Autodesk Inventor part; units mm, degrees
ref_plane "YZ Plane" through (0, 0, 0) normal (1, 0, 0) x (0, 1, 0)
ref_plane "XZ Plane" through (0, 0, 0) normal (0, 1, 0) x (-1, 0, 0)
ref_plane "XY Plane" through (0, 0, 0) normal (0, 0, 1) x (1, 0, 0)
sketch "Sketch1" plane through (0, 0, 0) normal (0, 0, 1) x (1, 0, 0)
  circle A0 centre (0, 0) radius 51
  dimension "d0" = 102
extrude "Extrusion1" add sketch "Sketch1" along normal blind 5
sketch "Sketch2" plane through (0, 0, 5) normal (0, 0, 1) x (1, 0, 0)
  point P0 (0, 0)
  point P1 (0, 0)
hole "Hole1" at (0, 0, 5) direction (0, 0, -1) diameter 6.6 depth 8 tip angle 118
sketch "Sketch3" plane through (0, 0, 5) normal (0, 0, 1) x (1, 0, 0)
  circle A0 centre (0, 0) radius 15 construction
  point P0 (-15, 0)
  point P1 (0, 15)
  point P2 (15, 0)
  point P3 (0, -15)
  dimension "d10" = 30
hole "Hole2" at (-15, 0, 5) at (0, 15, 5) at (15, 0, 5) at (0, -15, 5) direction (0, 0, -1) diameter 3.4 depth 8 tip angle 118
sketch "Sketch4" plane through (0, 0, 5) normal (0, 0, 1) x (1, 0, 0)
  line L0 (-51, 1.6) -> (-51, -1.6)
  line L1 (-51, -1.6) -> (-46, -1.6)
  line L2 (-46, -1.6) -> (-46, -2.75)
  line L3 (-46, -2.75) -> (-43.6, -2.75)
  line L4 (-43.6, -2.75) -> (-43.6, 2.75)
  line L5 (-43.6, 2.75) -> (-46, 2.75)
  line L6 (-46, 2.75) -> (-46, 1.6)
  line L7 (-46, 1.6) -> (-51, 1.6)
  line L8 (-1.6, -51) -> (1.6, -51)
  line L9 (1.6, -51) -> (1.6, -46)
  line L10 (1.6, -46) -> (2.75, -46)
  line L11 (2.75, -46) -> (2.75, -43.6)
  line L12 (2.75, -43.6) -> (-2.75, -43.6)
  line L13 (-2.75, -43.6) -> (-2.75, -46)
  line L14 (-2.75, -46) -> (-1.6, -46)
  line L15 (-1.6, -46) -> (-1.6, -51)
  line L16 (51, -1.6) -> (51, 1.6)
  line L17 (51, 1.6) -> (46, 1.6)
  line L18 (46, 1.6) -> (46, 2.75)
  line L19 (46, 2.75) -> (43.6, 2.75)
  line L20 (43.6, 2.75) -> (43.6, -2.75)
  line L21 (43.6, -2.75) -> (46, -2.75)
  line L22 (46, -2.75) -> (46, -1.6)
  line L23 (46, -1.6) -> (51, -1.6)
  line L24 (1.6, 51) -> (-1.6, 51)
  line L25 (-1.6, 51) -> (-1.6, 46)
  line L26 (-1.6, 46) -> (-2.75, 46)
  line L27 (-2.75, 46) -> (-2.75, 43.6)
  line L28 (-2.75, 43.6) -> (2.75, 43.6)
  line L29 (2.75, 43.6) -> (2.75, 46)
  line L30 (2.75, 46) -> (1.6, 46)
  line L31 (1.6, 46) -> (1.6, 51)
  point P0 (0, 0)
  point P1 (-43.6, 0)
  point P2 (-51, 0)
  point P3 (0, -51)
  point P4 (0, -43.6)
  point P5 (51, 0)
  point P6 (43.6, 0)
  point P7 (0, 51)
  point P8 (0, 43.6)
  dimension "d18" = 5.5
  dimension "d19" = 5
  dimension "d20" = 2.4
  dimension "d21" = 3.2
  dimension "d22" = 51
  dimension "d25" = 360
extrude "Extrusion2" cut sketch "Sketch4" against normal through all
equation "\"d27\" = d22"
properties part number "PlexiHalter2" material "Polycarbonate, Clear"
CAD build for the part. Positions are in the model's coordinates, mm. A direction names the side the tool comes from. Give positions to 0.01 mm unless a question says otherwise; leave off trailing zeros. Loops run counter-clockwise (first coordinate to the right, second up) from the corner with the lowest first, then second, coordinate; pieces in that order, holes last. Notation, with made-up numbers: (68.5, 39) - (116.5, 39) arc R21 ccw to (116.5, 72) - close; hole circle Ø9 at (42.25, -31). An arc over 180 degrees is marked (long way). Put each result on its own line as item: value.
Q1. Mould opens along X. For faces 1 (the face through (-36.44, 35.68, 2.46)), 2 (the face through (2.75, 45, 3)), 3 (the face through (48, -1.6, 3)) say: pulls with the +X half, pulls with the -X half, needs draft (parallel to the pull), parting line crosses it, or undercut.
Filled in:
face 1: pulls with the -X half
face 2: undercut
face 3: needs draft
Q2. Slice it at C-C (y = 15). Give the cut face in (x, z).
Filled in:
outline: (-48.74, 0) - (-1.7, 0) - (-1.7, 5) - (-48.74, 5) - close; (1.7, 0) - (48.74, 0) - (48.74, 5) - (1.7, 5) - close
Q3. Tool access for faces 4 (the face through (-49, -1.6, 3)), 5 (the face through (1.6, 48, 3)), 6 (the face through (1.6, -49, 3)), 7 (the face through (43.6, 0, 3)): list every direction of +Z, -Z, +X, -X, +Y, -Y with a clear straight run to the whole face (end or side of a thin tool).
Filled in:
face 4: +Z, -Z, -X
face 5: +Z, -Z, +Y
face 6: +Z, -Z, -Y
face 7: +Z, -Z
Q4. Slice it at A-A (x = 0). Give the cut face in (y, z), plus the area to 3 significant figures.
Filled in:
outline: (-43.6, 0) - (-16.7, 0) - (-16.7, 5) - (-43.6, 5) - close; (-13.3, 0) - (-3.3, 0) - (-3.3, 5) - (-13.3, 5) - close; (3.3, 0) - (13.3, 0) - (13.3, 5) - (3.3, 5) - close; (16.7, 0) - (43.6, 0) - (43.6, 5) - (16.7, 5) - close
area: 369 mm²
Q5. Flat gauge pins, fed straight in: pin 1 (3 mm diameter, centred on y = 25.5, z = 4.5, fed in from -X); pin 2 (1 mm diameter, centred on y = 20.5, z = 2.5, fed in from -X); pin 3 (1.5 mm diameter, centred on y = -47.5, z = 3.5, fed in from +X); pin 4 (2 mm diameter, centred on x = 0, y = -15, fed in from -Z). Where does each tip first touch, or does it go through?
Filled in:
pin 1: stops at x = -45
pin 2: stops at x = -46.91
pin 3: stops at x = 20.38
pin 4: passes through
Q6. Probe line 1 along Y through (x, z) = (0, 3.5); line 2 along X through (y, z) = (1.5, 0.3). List the from-to ranges inside material, lowest first.
Filled in:
line 1: y = -43.6 to -16.7, -13.3 to -3.3, 3.3 to 13.3, 16.7 to 43.6
line 2: x = -43.6 to -15.8, -14.2 to -2.94, 2.94 to 14.2, 15.8 to 43.6
